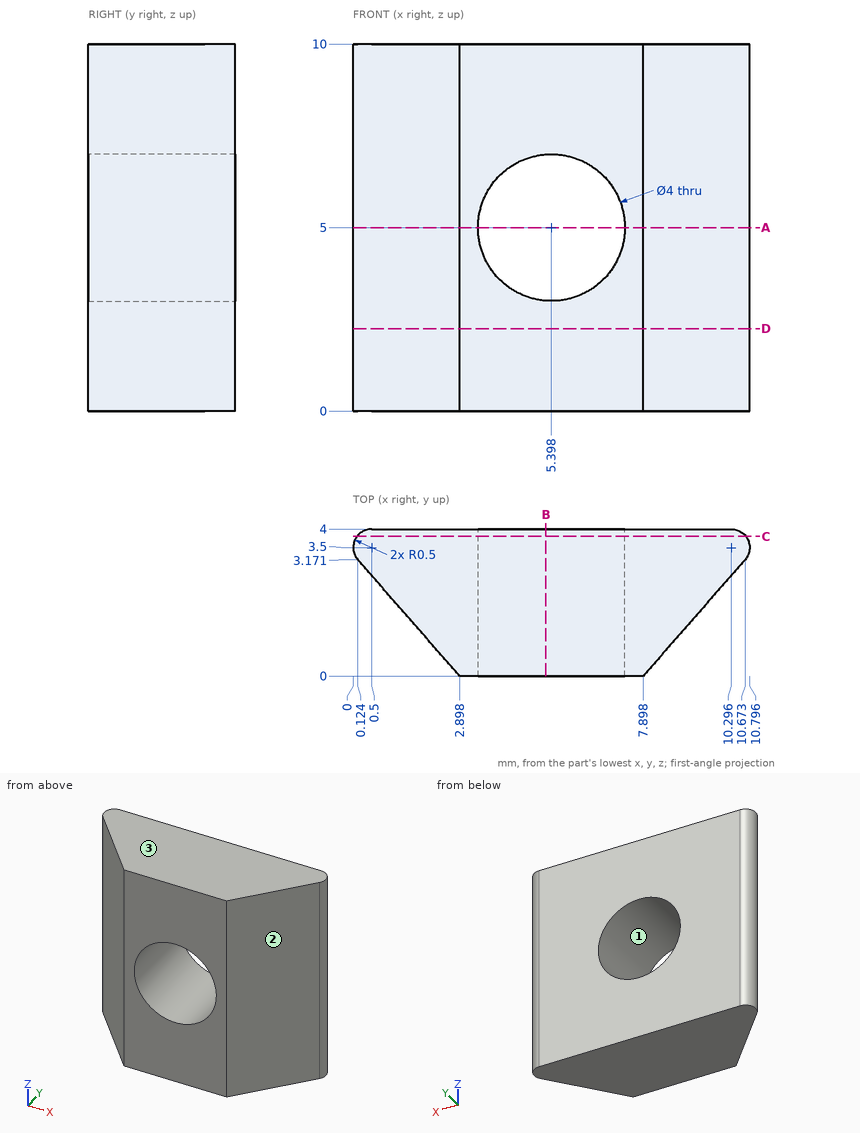
Part print with two shaded views. Sizes in mm from the minimum x, y, z corner. Coordinates: 2 decimals unless noted, no trailing zeros. Loops run counter-clockwise (first coordinate to the right, second up) from the corner with the lowest first, then second, coordinate; pieces in that order, holes last. Notation, with made-up numbers: (83.5, 20.25) - (141.5, 20.25) arc R24 cw to (141.5, 40.25) - close; hole circle Ø10 at (33.5, 62.5). An arc over 180 degrees is marked (long way). Write each question's results on one line, items separated by ' | '. Start each with the question number.
Q1. Two-plate mould, pull along X, no slides. Class the marked faces 1, 2 and 3: +X half, -X half, draft (parallel to the pull), parting line (faces both ways), or undercut.
Q2. Slice it at C-C on y = 3.8. Give the cut face in (x, z).
Q3. Probe line 1 along X through (y, z) = (0.95, 5) (1 decimal); line 2 along X through (y, z) = (1, 5) (1 decimal); line 3 along Z through (x, y) = (4.75, 3.1). List the from-to ranges inside material, lowest first.
Q4. Slice it at A-A on z = 5. Give the cut face in (x, y).
Q5. Slice it at B-B on x = 5.25. Give the cut face in (y, z) (1 decimal).
Q6. Slice it at D-D on z = 2.25. Give the cut face in (x, y).
Q7. Drop flat-ended pins along their axis: pin 1 Ø1.5 at (y, z) = (2, 2.5) entering from +X (1 decimal); pin 2 Ø2.5 at (x, z) = (5.4, 5) entering from +Y. Give the stop position or say it passes through.
Answer:
1) face 1: undercut | face 2: +X half | face 3: draft
2) outline: (0.1, 0) - (10.7, 0) - (10.7, 10) - (0.1, 10) - close; hole circle Ø4 at (5.4, 5)
3) line 1: x = 2.1 to 3.4, 7.4 to 8.7 | line 2: x = 2 to 3.4, 7.4 to 8.8 | line 3: z = 0 to 3.11, 6.89 to 10
4) outline: (0.12, 3.17) - (2.9, 0) - (3.4, 0) - (3.4, 4) - (0.5, 4) arc R0.5 ccw to start; (7.4, 0) - (7.9, 0) - (10.67, 3.17) arc R0.5 ccw to (10.3, 4) - (7.4, 4) - close
5) outline: (0, 0) - (4, 0) - (4, 3) - (0, 3) - close; (0, 7) - (4, 7) - (4, 10) - (0, 10) - close
6) outline: (0.12, 3.17) - (2.9, 0) - (7.9, 0) - (10.67, 3.17) arc R0.5 ccw to (10.3, 4) - (0.5, 4) arc R0.5 ccw to start
7) pin 1: stops at x = 10.3 | pin 2: passes through
